Here's how the part is built. I have some questions about the finished solid (model axes, mm). A direction names the side the tool comes from. Give positions to 0.01 mm unless a question says otherwise; leave off trailing zeros. Loops run counter-clockwise (first coordinate to the right, second up) from the corner with the lowest first, then second, coordinate; pieces in that order, holes last.
Q1. I'm going to push flat-ended pins straight in: P1, Ø8, axis at y = 60, z = 123.5, coming from the -X side; P2, Ø9, axis at y = 63.5, z = 20.5, coming from the +X side; P3, Ø12, axis at x = -72, z = 60, coming from the +Y side; P4, Ø9, axis at y = 63, z = 12.5, coming from the -X side. Where does each tip first touch, or does it pass through?
Q2. Suppose I cut it at B-B (z = 13.5). List the corners of the cut face in (x, y) for me.
Q3. Suppose I cut it at C-C (y = 74.5). List the corners of the cut face in (x, z) for me, and give its area (3 significant figures).
Q4. Thinking about a two-plate mould opening in Y: for faces 1 (the face through (-7.64, 119.76, 24.47)), 2 (the face through (-76.2, 63, 24)), 3 (the face through (-254, 37, 24)), which applies, pulls with the +Y half, pulls with the -Y half, needs draft (parallel to the pull), parting line crosses it, or undercut?
Q5. I need wall thicknesses on probe 1 along X at (y, z) = (79.5, 101); probe 2 along Y at (x, z) = (-67, 12); probe 3 along X at (y, z) = (64, 37). Which ranges of each line are inside material? Lowest first, please.
Q6. Suppose I cut it at A-A (x = -189). List the corners of the cut face in (y, z) for me.
Q7. For faces 4 (the face through (-170, 64, 48.26)), 5 (the face through (-85, 64, 48.26)), 6 (the face through (-38, 48.26, 24)), 7 (the face through (-215, 48.26, 24)), 8 (the face through (-246.36, 119.76, 24.47)), which set-ups out of +Z, -Z, +X, -X, +Y, -Y let a thin tool reach every point of the face, with its end or its side?
```python
from build123d import *

# Parameters (mm, degrees)
F1_DEPTH = 48.26
F3_DEPTH = 101.6
F4_R     = 63.49999
F5_R     = 25.4


# Not quite as in the source:
# - a fillet or chamfer is up to 0.001 mm smaller than in the source, because OpenCascade refuses the exact size
# - a feature names something its author has since deleted; it is built from what else it names


with BuildPart() as f1:
    # F0 (on Top) → F1 (new body)
    with BuildSketch(Plane.XY):
        Polygon((-254, 0), (0, 0), (0, 48.26), (-76.2, 48.26), (-76.2, 78.74), (0, 78.74), (0, 127), (-101.6, 127), (-152.4, 127), (-254, 127), (-254, 78.74), (-177.8, 78.74), (-177.8, 48.26), (-254, 48.26), align=None)
    extrude(amount=F1_DEPTH)

    # F2 (on face) → F3 (join)
    with BuildSketch(Plane.XY.offset(48.26)):
        Polygon((-101.6, 127), (-127, 127), (-152.4, 127), (-152.4, 0), (-101.6, 0), align=None)
    extrude(amount=F3_DEPTH)

    # F4 (radius 63.5 in the source; OpenCascade refuses exactly that, so slightly less here)
    f4_edges = [f1.edges().sort_by_distance(p)[0] for p in [
        (-127, 0, 149.86),
        (-127, 127, 149.86),
    ]]
    fillet(f4_edges, radius=F4_R)

    # F5
    f5_edges = [f1.edges().sort_by_distance(p)[0] for p in [
        (-254, 0, 24.13),
        (0, 0, 24.13),
        (-254, 127, 24.13),
        (0, 127, 24.13),
    ]]
    fillet(f5_edges, radius=F5_R)


solid = f1.part
```
Solutions:
1. P1: stops at x = -152.4
1. P2: stops at x = -76.2
1. P3: passes through
1. P4: stops at x = -177.8
2. outline: (-254, 25.4) arc R25.4 ccw to (-228.6, 0) - (-25.4, 0) arc R25.4 ccw to (0, 25.4) - (0, 48.26) - (-76.2, 48.26) - (-76.2, 78.74) - (0, 78.74) - (0, 101.6) arc R25.4 ccw to (-25.4, 127) - (-228.6, 127) arc R25.4 ccw to (-254, 101.6) - (-254, 78.74) - (-177.8, 78.74) - (-177.8, 48.26) - (-254, 48.26) - close
3. outline: (-177.8, 0) - (-76.2, 0) - (-76.2, 48.26) - (-101.6, 48.26) - (-101.6, 148.9) - (-152.4, 148.9) - (-152.4, 48.26) - (-177.8, 48.26) - close
3. area: 10,000 mm2
4. face 1: pulls with the +Y half
4. face 2: undercut
4. face 3: needs draft
5. probe 1: x = -152.4 to -101.6
5. probe 2: y = 0 to 48.26, 78.74 to 127
5. probe 3: x = -177.8 to -76.2
6. outline: (0, 0) - (48.26, 0) - (48.26, 48.26) - (0, 48.26) - close; (78.74, 0) - (127, 0) - (127, 48.26) - (78.74, 48.26) - close
7. face 4: +Z, -X, +Y, -Y
7. face 5: +Z, +X, +Y, -Y
7. face 6: +Z, -Z, +X
7. face 7: +Z, -Z, -X
7. face 8: +Z, -Z, -X, +Y
